For this review, take the finished solid that the model builds, in its own axes (mm). Coordinates: 2 decimals unless noted, no trailing zeros. Order: outer loops, then holes, each group sorted by start corner. A loop starts at its lowest first (then second) coordinate and runs counter-clockwise, first axis right, second up. Notation, with made-up numbers: (78.5, 53) -> (83.5, 53) arc R27 ccw to (83.5, 73) -> close; hole circle Ø6 at (57, -16). An arc over 180 degrees is marked (long way). Write item = value, one per line. Start each with the question number.
1) Consider section D-D on x = -133.5. Give the boundary of the cut face in (y, z).
2) Consider section C-C on z = 89. Give the boundary of the cut face in (x, y), and give its area (3 significant figures).
3) Wall thickness on probe 1 along X at (y, z) = (1, 72); probe 2 along Y at (x, z) = (-49, 42.5); probe 3 along X at (y, z) = (9, 40.5): over which ranges is each line inside the solid? List them lowest first. Write a range as [from, to].
4) Consider section A-A on x = -4. Give the boundary of the cut face in (y, z), and give its area (3 significant figures).
5) Insertion check: pin 1 Ø3 at (x, y) = (-6.5, 7.5) entering from -Z; pin 2 Ø1 at (y, z) = (1, 14) entering from +X; pin 3 Ø8 at (x, y) = (-104.5, 2.5) entering from -Z; pin 4 Ø10 at (x, z) = (-177, 87.5) entering from +Y. Each pin has a flat end and moves straight along its axis. Give the tip position at first contact, or say it passes through.
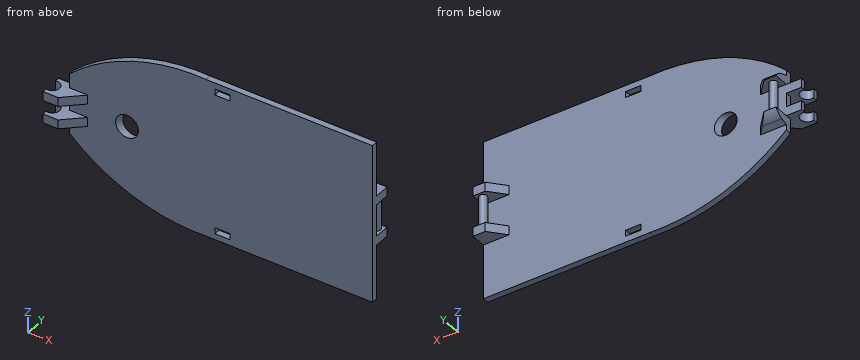
from build123d import *
from OCP.BRepFilletAPI import BRepFilletAPI_MakeChamfer

# Parameters (mm, degrees)
BOSS_EXTRUDE1_DEPTH  = 4
BOSS_EXTRUDE2_START  = -45
BOSS_EXTRUDE2_DEPTH  = 3
BOSS_EXTRUDE3_START  = -39
BOSS_EXTRUDE3_DEPTH  = 3
BOSS_EXTRUDE4_REACH  = 221.731
SKETCH6_R            = 2.5
SKETCH7_W            = 10
SKETCH7_H            = 4
CUT_EXTRUDE1_DEPTH   = 10
SKETCH8_R            = 7.5
MIRROR6_START        = -39
MIRROR6_COPY_1_DEPTH = 3
CHAMFER1_SIZE        = 10
CHAMFER1_SIZE_2      = 3.249196962
FILLET1_R            = 10
SKETCH10_R           = 2.5
BOSS_EXTRUDE6_DEPTH  = 23


# Some blends are built 0.0001 mm under size
with BuildPart() as part:
    # Sketch1 → Boss-Extrude1 (new body)
    with BuildSketch(Plane(origin=(0, 0, 0), x_dir=(1, 0, 0), z_dir=(0, 1, 0))):
        with BuildLine():
            Line((-110, 0), (0, 0))
            Line((0, 0), (0, -105))
            Line((0, -105), (-110, -105))
            ThreePointArc((-110, -105), (-158.232963684, -97.702822508), (-200, -72.5))
            Line((-200, -72.5), (-200, -32.5))
            ThreePointArc((-200, -32.5), (-158.232963684, -7.297177492), (-110, 0))
        make_face()
    extrude(amount=BOSS_EXTRUDE1_DEPTH)

    # Sketch2 → Boss-Extrude2 (add, symmetric)
    with BuildSketch(Plane.XY.offset(105).offset(BOSS_EXTRUDE2_START)):
        with BuildLine():
            Line((-200, 4), (-210, 4))
            Line((-210, 4), (-210, 1))
            ThreePointArc((-210, 1), (-204.2, -3.5), (-210, -8))
            Line((-210, -8), (-210, -11))
            Line((-210, -11), (-200, -11))
            Line((-200, -11), (-188, 0))
            Line((-188, 0), (-200, 4))
        make_face()
    boss_extrude2 = extrude(amount=BOSS_EXTRUDE2_DEPTH, both=True)

    # Mirror1: Boss-Extrude2 across plane
    add(boss_extrude2.mirror(Plane.XY.offset(52.5)))

    # Sketch5 → Boss-Extrude3 (add, symmetric)
    with BuildSketch(Plane.XY.offset(105).offset(BOSS_EXTRUDE3_START)):
        Polygon((-16.979807258, 4), (-7.979807258, 14), (0, 14), (0, 4), align=None)
    boss_extrude3 = extrude(amount=BOSS_EXTRUDE3_DEPTH, both=True)

    # Mirror4: Boss-Extrude3 across plane
    add(boss_extrude3.mirror(Plane.XY.offset(52.5)))

    # Sketch6 → Boss-Extrude4 (add, up to next)
    with BuildSketch(Plane.XY.offset(42), mode=Mode.PRIVATE) as boss_extrude4_sk1:
        with Locations(Location((-4, 10, 0), (0, 0, 180))):
            Circle(SKETCH6_R)
    boss_extrude4_tool1 = extrude(boss_extrude4_sk1.sketch, amount=BOSS_EXTRUDE4_REACH, mode=Mode.PRIVATE) - part.part
    add(boss_extrude4_tool1.solids().sort_by_distance((-4, 10, 42))[0])

    # Sketch7 → Cut-Extrude1 (cut)
    with BuildSketch(Plane(origin=(0, 4, 0), x_dir=(1, 0, 0), z_dir=(0, 1, 0))):
        with Locations((-99, -99)):
            Rectangle(SKETCH7_W, SKETCH7_H)
    cut_extrude1 = extrude(amount=-CUT_EXTRUDE1_DEPTH, mode=Mode.SUBTRACT)

    # Mirror5: Cut-Extrude1 across plane
    add(cut_extrude1.mirror(Plane.XY.offset(52.5)), mode=Mode.SUBTRACT)

    # Cut-Sweep1: sweep along a path in Sketch9
    with BuildLine(Plane.XY.offset(52.5)) as cut_sweep1_path:
        Line((-160, 4), (-163.867437875, -3.466183031))
    # Sketch8 → Cut-Sweep1 (sweep, cut)
    with BuildSketch(Plane(origin=(0, 4, 0), x_dir=(1, 0, 0), z_dir=(0, 1, 0))):
        with Locations((-160, -52.5)):
            Circle(SKETCH8_R)
    sweep(path=cut_sweep1_path.line, mode=Mode.SUBTRACT)

    # Mirror6: Boss-Extrude3 across plane
    add(boss_extrude3.mirror(Plane(origin=(-100, 0, 0), x_dir=(0, 0, 1), z_dir=(1, 0, 0))))

    # Mirror6 copy 1 sketch → Mirror6 copy 1 (add, symmetric)
    with BuildSketch(Plane(origin=(-200, 0, 0), x_dir=(-1, 0, 0), z_dir=(0, 0, -1)).offset(MIRROR6_START)):
        Polygon((-16.979807258, 4), (-7.979807258, 14), (0, 14), (0, 4), align=None)
    extrude(amount=MIRROR6_COPY_1_DEPTH, both=True)

    # Chamfer1
    chamfer1_edges_1 = [part.edges().sort_by_distance(p)[0] for p in [
        (-196.010096371, 14, 69),
    ]]
    chamfer1_side_1 = [part.faces().sort_by_distance(p)[0] for p in [
        (-196.010096371, 13.935016061, 69),
    ]]
    chamfer1_edges_2 = [part.edges().sort_by_distance(p)[0] for p in [
        (-196.010096371, 14, 36),
    ]]
    chamfer1_side_2 = [part.faces().sort_by_distance(p)[0] for p in [
        (-196.010096371, 13.935016061, 36),
    ]]
    chamfer1 = BRepFilletAPI_MakeChamfer(part.part.solid().wrapped)
    for e in chamfer1_edges_1:
        chamfer1.Add(CHAMFER1_SIZE - 0.0001, CHAMFER1_SIZE_2 - 0.0001, e.wrapped, chamfer1_side_1[0].wrapped)
    for e in chamfer1_edges_2:
        chamfer1.Add(CHAMFER1_SIZE - 0.0001, CHAMFER1_SIZE_2 - 0.0001, e.wrapped, chamfer1_side_2[0].wrapped)
    add(Compound.cast(chamfer1.Shape()), mode=Mode.REPLACE)  # a hair under: the kernel refuses the full size

    # Fillet1
    # the kernel refuses this fillet: 10 mm, written as the material it takes off along each edge
    with BuildSketch(Plane(origin=(-177.285530003, 14, 39.249096962), x_dir=(0, 0, 1), z_dir=(-1, 0, 0))) as fillet1_piece_1:
        with BuildLine():
            CenterArc((7.689313783, -8.695521796), FILLET1_R, 119.593358477, 42.406991386)
            Line((-1.821270249, -5.605409927), (-2.01148193, -5.543607689))
            Line((-2.01148193, -5.543607689), (-0.190211681, 0.061802237))
            Line((-0.190211681, 0.061802237), (0, 0.2))
            ThreePointArc((0, 0.2), (1.375451519, 0.2), (2.652134823, 0.173910436))
            Line((2.652134823, 0.173910436), (2.750903038, 0))
        make_face()
    extrude(amount=37.449132737, mode=Mode.SUBTRACT)
    with BuildSketch(Plane(origin=(-177.285530003, 14, 65.750903038), x_dir=(0, 0, -1), z_dir=(-1, 0, 0))) as fillet1_piece_2:
        with BuildLine():
            CenterArc((7.689313783, 8.695521796), FILLET1_R, 197.999650137, 42.406991386)
            Line((-1.821270249, 5.605409927), (-2.01148193, 5.543607689))
            Line((-2.01148193, 5.543607689), (-0.190211681, -0.061802237))
            Line((-0.190211681, -0.061802237), (0, -0.2))
            ThreePointArc((0, -0.2), (1.375451519, -0.2), (2.652134823, -0.173910436))
            Line((2.652134823, -0.173910436), (2.750903038, 0))
        make_face()
    extrude(amount=37.449132737, mode=Mode.SUBTRACT)

    # Sketch10 → Boss-Extrude6 (add)
    with BuildSketch(Plane.XY.offset(42)):
        with Locations(Location((-195, 9, 0), (0, 0, 180))):
            Circle(SKETCH10_R)
    extrude(amount=BOSS_EXTRUDE6_DEPTH)


solid = part.part
Answer sheet:
q1.outline = (0, 1.13) -> (4, 1.13) -> (4, 103.87) -> (0, 103.87) -> close
q2.outline = (-177.2, 0) -> (0, 0) -> (0, 4) -> (-177.2, 4) -> close
q2.area = 709 mm2
q3.probe_1 = [-200, 0]
q3.probe_2 = [0, 4]
q3.probe_3 = [-200, -187.52], [-12.48, 0]
q4.outline = (0, 0) -> (4, 0) -> (4, 36) -> (14, 36) -> (14, 42) -> (12.5, 42) -> (12.5, 63) -> (14, 63) -> (14, 69) -> (4, 69) -> (4, 105) -> (0, 105) -> close; hole (4, 42) -> (7.5, 42) -> (7.5, 63) -> (4, 63) -> close
q4.area = 645 mm2
q5.pin_1 = 36
q5.pin_2 = 0
q5.pin_3 = 0
q5.pin_4 = 4
